Read the model definition and answer for the solid it produces. Units are mm, in the model's axes. Face numbers are marked on the shaded views. A direction names the side the tool comes from. Coordinates: 2 decimals unless noted, no trailing zeros. Write each loop counter-clockwise with the first axis right and the second up, starting at its lowest first coordinate (ties: lowest second). Pieces come first, ordered by that corner, then holes.
1) The part is cut by section A-A (x = 0). Determine the outline of the cut face in (y, z) (3 decimals), then the cut area to 3 significant figures.
2) Determine the mould class of the marked faces 1, 2 and 3 for opening direction Y: +Y half, -Y half, draft (parallel to the pull), parting line (faces both ways), or undercut.
3) Find the intervals of material crossed by line 1 (Z direction, x = -17, y = -11.5); line 2 (Y direction, x = 0, z = 10.25) (3 decimals); line 3 (X direction, y = 1, z = 7.5), in increasing order.
4) Which of the six approach directions +Z, -Z, +X, -X, +Y, -Y give full straight-line access (tool end or side, diameter ignored) to the marked faces 4 and 5?
5) The part is cut by section D-D (y = -9.5). Determine the outline of the cut face in (x, z).
6) Each of these flat-tipped pins is pushed along its axis until it touches: pin 1 Ø1.5 at (x, z) = (-15, 7.5) entering from -Y; pin 2 Ø9.5 at (x, y) = (0, 0) entering from -Z; pin 3 Ø2 at (y, z) = (-16, 18) entering from +X; pin 4 Ø3 at (y, z) = (9, 6.5) entering from -X. Where does it stop, or does it pass through?
7) The part is cut by section C-C (z = 7.75). Determine the outline of the cut face in (x, y) (3 decimals), then the cut area to 3 significant figures.
8) The part is cut by section B-B (y = 0). Determine the outline of the cut face in (x, z) (3 decimals).
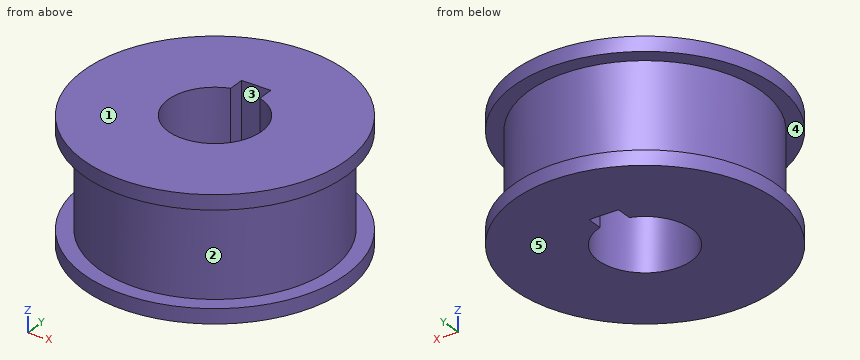
Autodesk Inventor part; units mm, degrees
ref_plane "YZ Plane" through (0, 0, 0) normal (1, 0, 0) x (0, 1, 0)
ref_plane "XZ Plane" through (0, 0, 0) normal (0, 1, 0) x (-1, 0, 0)
ref_plane "XY Plane" through (0, 0, 0) normal (0, 0, 1) x (1, 0, 0)
sketch "Sketch1" plane through (0, 0, 0) normal (0, 0, 1) x (1, 0, 0)
  circle A0 centre (0, 0) radius 22.5
  dimension "d0" = 45
extrude "Extrusion1" add sketch "Sketch1" along normal blind 2.5
sketch "Sketch2" plane through (0, 0, 2.5) normal (0, 0, 1) x (1, 0, 0)
  circle A0 centre (0, 0) radius 19.895
  dimension "d3" = 39.79
extrude "Extrusion2" add sketch "Sketch2" along normal blind 16
sketch "Sketch3" plane through (0, 0, 18.5) normal (0, 0, 1) x (1, 0, 0)
  circle A0 centre (0, 0) radius 22.5
  dimension "d6" = 45
extrude "Extrusion3" add sketch "Sketch3" along normal blind 2.5
sketch "Sketch4" plane through (0, 0, 21) normal (0, 0, 1) x (1, 0, 0)
  circle A0 centre (0, 0) radius 8
  line L0 (-2.5, 5.7) -> (2.5, 5.7)
  line L1 (2.5, 5.7) -> (2.5, 10.3)
  line L2 (2.5, 10.3) -> (-2.5, 10.3)
  line L3 (-2.5, 10.3) -> (-2.5, 5.7)
  line L4 (-2.5, 5.7) -> (2.5, 10.3) construction
  line L5 (2.5, 5.7) -> (-2.5, 10.3) construction
  point P0 (0, 8)
  dimension "d9" = 16
  dimension "d10" = 5
  dimension "d11" = 4.6
extrude "Extrusion4" cut sketch "Sketch4" against normal blind 21
properties part number "HTD5M 25 Pulley" material "Aluminum 6061"
Reported:
1. outline: (-22.5, 0) - (-8, 0) - (-8, 21) - (-22.5, 21) - (-22.5, 18.5) - (-19.895, 18.5) - (-19.895, 2.5) - (-22.5, 2.5) - close; (10.3, 0) - (22.5, 0) - (22.5, 2.5) - (19.895, 2.5) - (19.895, 18.5) - (22.5, 18.5) - (22.5, 21) - (10.3, 21) - close
1. area: 477 mm2
2. face 1: draft
2. face 2: parting line
2. face 3: undercut
3. line 1: z = 0 to 2.5, 18.5 to 21
3. line 2: y = -19.895 to -8, 10.3 to 19.895
3. line 3: x = -19.87 to -7.94, 7.94 to 19.87
4. face 4: none
4. face 5: -Z, +X, -X, +Y, -Y
5. outline: (-20.4, 0) - (20.4, 0) - (20.4, 2.5) - (17.48, 2.5) - (17.48, 18.5) - (20.4, 18.5) - (20.4, 21) - (-20.4, 21) - (-20.4, 18.5) - (-17.48, 18.5) - (-17.48, 2.5) - (-20.4, 2.5) - close
6. pin 1: stops at y = -13.88
6. pin 2: passes through
6. pin 3: stops at x = 16.65
6. pin 4: stops at x = -18.43
7. outline: circle Ø39.79 at (0, 0); hole (-2.5, 7.599) arc R8 ccw (long way) to (2.5, 7.599) - (2.5, 10.3) - (-2.5, 10.3) - close
7. area: 1,030 mm2
8. outline: (-22.5, 0) - (-8, 0) - (-8, 21) - (-22.5, 21) - (-22.5, 18.5) - (-19.895, 18.5) - (-19.895, 2.5) - (-22.5, 2.5) - close; (8, 0) - (22.5, 0) - (22.5, 2.5) - (19.895, 2.5) - (19.895, 18.5) - (22.5, 18.5) - (22.5, 21) - (8, 21) - close
